Geometry check sheet. Reference: drawing and pictorial views, mm from the part's lowest x, y, z. A direction names the side the tool comes from. Coordinates: 2 decimals unless noted, no trailing zeros. Loops run counter-clockwise (first coordinate to the right, second up) from the corner with the lowest first, then second, coordinate; pieces in that order, holes last. Notation, with made-up numbers: M 8,13 L 36,13 A22 ccw 36,49 Z; hole C -14.5,44 d4. An arc over 180 degrees is marked long. Write item = value, one per line. Start each with the question number.
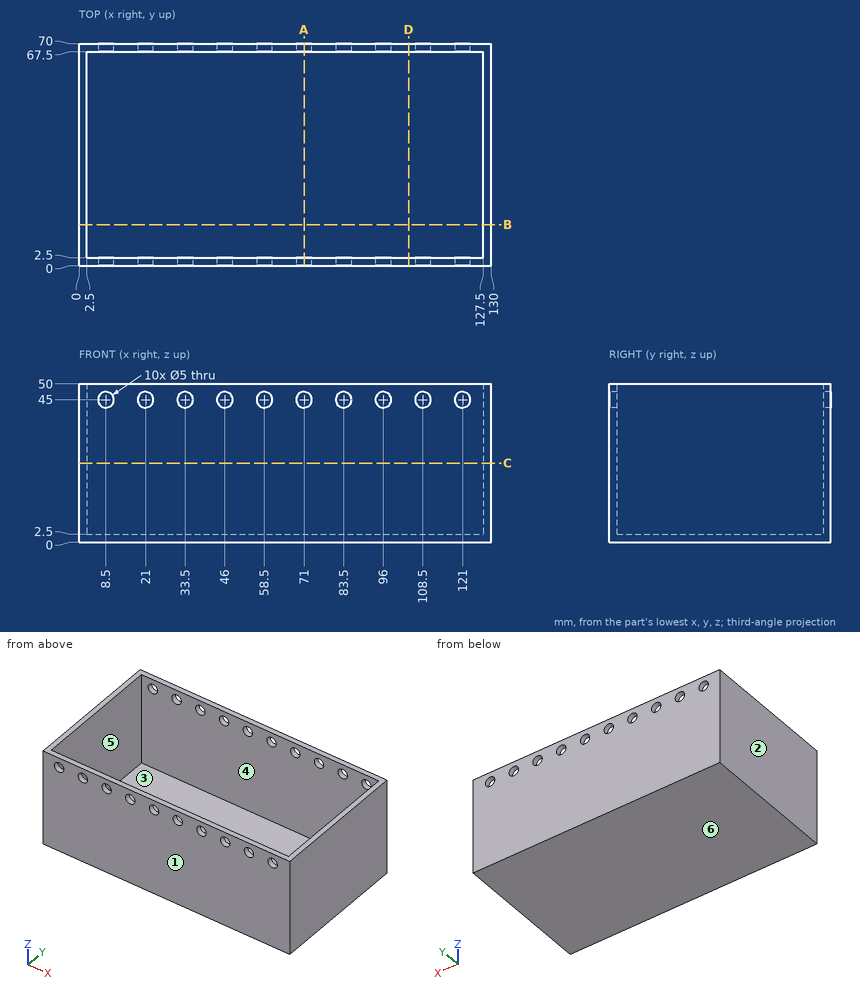
Q1. Sectioned sample at D-D on x = 104. Record the cut outline in (y, z).
Q2. Sectioned sample at B-B on y = 13. Record the cut outline in (x, z).
Q3. Scan lines: L1, parallel to Y at x = 81, z = 16.5; L2, parallel to X at y = 51, z = 17; L3, parallel to Z at x = 33.5, y = 69. Record each from-to range of solid material in increasing order. Write a range as [from, to].
Q4. Sectioned sample at A-A on x = 71. Record the cut outline in (y, z), plus the area to 4 significant figures.
Q5. Set-up check for the marked faces 5 and 6: record each of +Z, -Z, +X, -X, +Y, -Y from which the full face is reachable in a straight line by a thin tool's end or side.
Q6. Gauge pin test, flat ends, axial feed: pin 1 (8 mm diameter, centred on x = 77, y = 31, fed in from +Z); pin 2 (4.5 mm diameter, centred on x = 33.5, z = 45, fed in from +Y). Record the tip position at first contact, or that the pin passes through.
Q7. Sectioned sample at C-C on z = 25. Record the cut outline in (x, y).
Q8. Mould release check, pull along X, two halves, no side actions. Record for the marked faces 1, 2, 3 and 4: +X half, -X half, draft (parallel to the pull), parting line (faces both ways), or undercut.
Solutions:
q1.outline = M 0,0 L 70,0 L 70,50 L 67.5,50 L 67.5,2.5 L 2.5,2.5 L 2.5,50 L 0,50 Z
q2.outline = M 0,0 L 130,0 L 130,50 L 127.5,50 L 127.5,2.5 L 2.5,2.5 L 2.5,50 L 0,50 Z
q3.L1 = [0, 2.5], [67.5, 70]
q3.L2 = [0, 2.5], [127.5, 130]
q3.L3 = [0, 42.5], [47.5, 50]
q4.outline = M 0,0 L 70,0 L 70,42.5 L 67.5,42.5 L 67.5,2.5 L 2.5,2.5 L 2.5,42.5 L 0,42.5 Z; M 0,47.5 L 2.5,47.5 L 2.5,50 L 0,50 Z; M 67.5,47.5 L 70,47.5 L 70,50 L 67.5,50 Z
q4.area = 387.5 mm²
q5.face_5 = +Z
q5.face_6 = -Z, +X, -X, +Y, -Y
q6.pin_1 = 2.5
q6.pin_2 = through
q7.outline = M 0,0 L 130,0 L 130,70 L 0,70 Z; hole M 2.5,2.5 L 127.5,2.5 L 127.5,67.5 L 2.5,67.5 Z
q8.face_1 = draft
q8.face_2 = -X half
q8.face_3 = undercut
q8.face_4 = undercut
